Design review of the part built by this model. Coordinates are the model's own, in mm. Face numbers are marked on the shaded views. Coordinates: 2 decimals unless noted, no trailing zeros. Order: outer loops, then holes, each group sorted by start corner. A loop starts at its lowest first (then second) coordinate and runs counter-clockwise, first axis right, second up. Notation, with made-up numbers: (69.25, -19.5) -> (113.25, -19.5) arc R9 cw to (113.25, -15.5) -> close; hole circle Ø9 at (78.25, -7). An arc over 180 degrees is marked (long way). Use a Markdown table: item, result. Add a question column.
Q1. The part is to be moulded in two halves that separate along X. For the marked faces 1, 2 and 3, say which applies: pulls with the +X half, pulls with the -X half, needs draft (parallel to the pull), parting line crosses it, or undercut.
Q2. Insertion check: pin 1 (1 mm diameter, centred on x = -16.5, z = 7, fed in from +Y). The pin has a flat end and moves straight along its axis. Give the tip position at first contact, or say it passes through.
Q3. Add section C-C (x = 18.5). State the section outline as (y, z) points, then the cut area to 3 significant figures.
Q4. Wall thickness on probe 1 along Z at (x, y) = (-1, 6); probe 2 along X at (y, z) = (6.75, -32); probe 3 along Z at (x, y) = (-22.5, 0.75): over which ranges is each line inside the solid? List them lowest first.
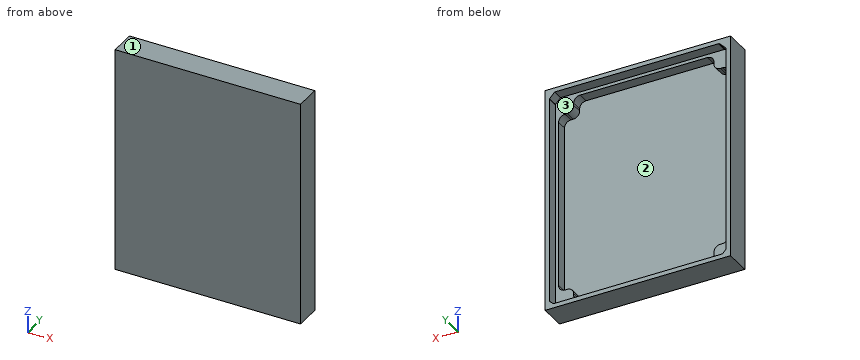
Autodesk Inventor part; units mm, degrees
ref_plane "YZ Plane" through (0, 0, 0) normal (1, 0, 0) x (0, 1, 0)
ref_plane "XZ Plane" through (0, 0, 0) normal (0, 1, 0) x (-1, 0, 0)
ref_plane "XY Plane" through (0, 0, 0) normal (0, 0, 1) x (1, 0, 0)
sketch "Sketch1" plane through (0, 0, 0) normal (0, 1, 0) x (-1, 0, 0)
  line L0 (41, 50.45) -> (40.9472, -50.4928) construction
  line L1 (40.9472, -50.4928) -> (-41, -50.45) construction
  line L2 (-41, -50.45) -> (-40.9472, 50.4928) construction
  line L3 (-40.9472, 50.4928) -> (41, 50.45) construction
  line L4 (-41, 50.45) -> (41, -50.45) construction
  line L5 (41, 50.45) -> (-41, -50.45) construction
  line L6 (-43, 52.45) -> (43, 52.45)
  line L7 (43, 52.45) -> (43, -52.45)
  line L8 (43, -52.45) -> (-43, -52.45)
  line L9 (-43, -52.45) -> (-43, 52.45)
  line L10 (-43, 52.45) -> (43, -52.45) construction
  line L11 (43, 52.45) -> (-43, -52.45) construction
  line L12 (41, 50.45) -> (41, 50.0105)
  line L13 (41.001, 46.9167) -> (41.001, -48.4427)
  line L14 (41, -50.45) -> (40.9473, -50.45)
  line L15 (39.0158, -50.4509) -> (-38.9625, -50.4509)
  line L16 (-38.3742, 50.45) -> (37.4278, 50.45)
  line L17 (-40.999, -48.5131) -> (-40.9487, 47.6278)
  line L18 (37.4278, 50.45) -> (37.7432, 50.4517)
  line L19 (41.001, 46.9167) -> (41.0014, 47.2908)
  line L20 (41.0014, 47.2908) -> (37.7432, 50.4517)
  line L21 (41.001, -48.4427) -> (41.001, -48.6823)
  line L22 (41.001, -48.6823) -> (39.229, -50.4509)
  line L23 (39.229, -50.4509) -> (39.0158, -50.4509)
  line L24 (-38.9625, -50.4509) -> (-39.191, -50.4509)
  line L25 (-39.191, -50.4509) -> (-40.9991, -48.7299)
  line L26 (-40.999, -48.5131) -> (-40.9991, -48.7299)
  line L27 (-40.9487, 47.6278) -> (-40.9486, 47.9339)
  line L28 (-38.3742, 50.45) -> (-38.6199, 50.45)
  line L29 (-38.6199, 50.45) -> (-40.9486, 47.9339)
  point P0 (0, 0)
  dimension "d48" = 82
  dimension "d49" = 100.9
  dimension "d50" = 86
  dimension "d51" = 104.9
extrude "Extrusion3" add sketch "Sketch1" along normal blind 10
sketch "Sketch3" plane through (0, 0, 0) normal (0, -1, 0) x (1, 0, 0)
  line L0 (43, -52.45) -> (-43, -52.45)
  line L1 (-43, 52.45) -> (43, 52.45)
  line L2 (43, 52.45) -> (43, -52.45)
  line L3 (43, -52.45) -> (-43, -52.45)
  line L4 (-43, -52.45) -> (-43, 52.45)
  line L5 (-43, 52.45) -> (43, -52.45) construction
  line L6 (43, 52.45) -> (-43, -52.45) construction
  point P0 (0, 0)
extrude "Extrusion4" add sketch "Sketch3" along normal blind 2
sketch "Sketch4" plane through (0, 0, 0) normal (0, 1, 0) x (1, 0, 0)
  line L0 (-40.966, -50.4517) -> (-40.966, 50.4509) construction
  line L1 (-40.966, 50.4509) -> (40.9486, 50.4509) construction
  line L2 (40.9486, 50.4509) -> (40.9486, -50.4517) construction
  line L3 (40.9486, -50.4517) -> (-40.966, -50.4517) construction
  line L4 (-41.001, -46.9167) -> (-41.001, 48.6823)
  line L5 (-37.7432, -50.4517) -> (-41.0014, -47.2908)
  line L6 (38.6199, -50.45) -> (-37.4278, -50.45)
  line L7 (43, 52.45) -> (-43, 52.45)
  line L8 (-43, 52.45) -> (-43, -52.45)
  line L9 (-43, -52.45) -> (43, -52.45)
  line L10 (43, -52.45) -> (43, 52.45)
  line L11 (-41.0014, -47.2908) -> (-41.001, -46.9167)
  line L12 (-41.001, -46.9167) -> (-41.001, 48.6823)
  line L13 (-41.001, 48.6823) -> (-39.229, 50.4509)
  line L14 (-39.229, 50.4509) -> (38.9625, 50.4509)
  line L15 (38.9625, 50.4509) -> (39.191, 50.4509)
  line L16 (39.191, 50.4509) -> (40.9991, 48.7299)
  line L17 (40.9991, 48.7299) -> (40.9486, -47.9339)
  line L18 (40.9486, -47.9339) -> (38.6199, -50.45)
  line L19 (38.6199, -50.45) -> (-37.4278, -50.45)
  line L20 (-37.4278, -50.45) -> (-37.7432, -50.4517)
  line L21 (-37.7432, -50.4517) -> (-41.0014, -47.2908)
  line L22 (-39.229, 50.4509) -> (38.9625, 50.4509)
  line L23 (-41.001, 48.6823) -> (-39.229, 50.4509)
  point P0 (0, 0)
sketch "Sketch5" plane through (0, 0, 0) normal (0, 1, 0) x (1, 0, 0)
  line L0 (-37.7432, -50.4517) -> (-41.0014, -47.2908)
  line L1 (-37.4278, -50.45) -> (-37.7432, -50.4517)
  line L2 (38.6199, -50.45) -> (-37.4278, -50.45)
  line L3 (40.9486, -47.9339) -> (38.6199, -50.45)
  line L4 (40.9991, 48.7299) -> (40.9486, -47.9339)
  line L5 (39.191, 50.4509) -> (40.9991, 48.7299)
  line L6 (38.9625, 50.4509) -> (39.191, 50.4509)
  line L7 (-39.229, 50.4509) -> (38.9625, 50.4509)
  line L8 (-41.001, 48.6823) -> (-39.229, 50.4509)
  line L9 (-41.001, -46.9167) -> (-41.001, 48.6823)
  line L10 (-41.0014, -47.2908) -> (-41.001, -46.9167)
  line L11 (-37.7432, -50.4517) -> (-41.0014, -47.2908)
  line L12 (38.6199, -50.45) -> (-37.4278, -50.45)
  line L13 (-37.4278, -50.45) -> (-37.7432, -50.4517)
  line L14 (-41.001, -46.9167) -> (-41.001, 48.6823)
  line L15 (-41.0014, -47.2908) -> (-41.001, -46.9167)
  line L16 (-41.001, 48.6823) -> (-39.229, 50.4509)
  line L17 (-39.229, 50.4509) -> (38.9625, 50.4509)
  line L18 (39.191, 50.4509) -> (40.9991, 48.7299)
  line L19 (40.9991, 48.7299) -> (40.9486, -47.9339)
  line L20 (40.9486, -47.9339) -> (38.6199, -50.45)
  line L21 (-41.0014, -47.2908) -> (-40.9669, 48.7164)
  line L22 (-39.229, 50.4509) -> (39.191, 50.4509)
  line L23 (40.9485, 48.778) -> (40.9486, -47.9339)
  line L24 (38.6199, -50.45) -> (-37.7432, -50.4517)
  line L25 (-37.7432, -50.4517) -> (-41.0014, -47.2908)
  line L26 (39.5283, -48.9788) -> (-39.5283, -48.9788)
  line L27 (-39.5283, -48.9788) -> (-39.5283, 48.9788)
  line L28 (-39.5283, 48.9788) -> (39.5283, 48.9788)
  line L29 (39.5283, 48.9788) -> (39.5283, -48.9788)
  line L30 (39.5283, -48.9788) -> (-39.5283, 48.9788) construction
  line L31 (-39.5283, -48.9788) -> (39.5283, 48.9788) construction
  line L32 (-39.5283, -48.9788) -> (-32.5283, -48.9788)
  line L33 (-32.5283, -48.9788) -> (-32.5283, -41.9788)
  line L34 (-32.5283, -41.9788) -> (-39.5283, -41.9788)
  line L35 (-39.5283, -41.9788) -> (-39.5283, -48.9788)
  line L36 (-39.5283, 48.9788) -> (-32.5283, 48.9788)
  line L37 (-32.5283, 48.9788) -> (-32.5283, 41.9788)
  line L38 (-32.5283, 41.9788) -> (-39.5283, 41.9788)
  line L39 (-39.5283, 41.9788) -> (-39.5283, 48.9788)
  line L40 (39.5283, 48.9788) -> (32.5283, 48.9788)
  line L41 (32.5283, 48.9788) -> (32.5283, 41.9788)
  line L42 (32.5283, 41.9788) -> (39.5283, 41.9788)
  line L43 (39.5283, 41.9788) -> (39.5283, 48.9788)
  line L44 (39.5283, -48.9788) -> (32.5283, -48.9788)
  line L45 (32.5283, -48.9788) -> (32.5283, -41.9788)
  line L46 (32.5283, -41.9788) -> (39.5283, -41.9788)
  line L47 (39.5283, -41.9788) -> (39.5283, -48.9788)
  point P0 (0, 0)
  point P1 (-41.001, -46.1517)
  point P2 (-39.5283, -48.7199)
  point P3 (-39.2615, -48.9788)
  dimension "d152" = 7
  dimension "d153" = 7
  dimension "d154" = 7
  dimension "d155" = 7
  dimension "d156" = 7
  dimension "d157" = 7
  dimension "d158" = 7
  dimension "d159" = 7
extrude "Extrusion5" add sketch "Sketch5" along normal blind 5 contours L0 L26 L29 L28 L27 L10 L21 L8 L7 L6 L5 L23 L3 L2 L1 | L0 L27 L34 L33 L26 | L45 L46 L29 L26 | L27 L28 L37 L38 | L42 L41 L28 L29
fillet "Fillet1" radius 3 12 edges at (-39.5283, 2.5, 41.9788) (-32.5283, 2.5, 41.9788) (-32.5283, 2.5, 48.9788) (-32.5283, 2.5, -48.9788) (-32.5283, 2.5, -41.9788) (-39.5283, 2.5, -41.9788) (32.5283, 2.5, -48.9788) (32.5283, 2.5, -41.9788) (39.5283, 2.5, -41.9788) (39.5283, 2.5, 41.9788) (32.5283, 2.5, 41.9788) (32.5283, 2.5, 48.9788)
properties part number "box"
Established:
| question | item | result |
|---|---|---|
| 1 | face 1 | needs draft |
| 1 | face 2 | undercut |
| 1 | face 3 | undercut |
| 2 | pin 1 | y = 0 |
| 3 | outline | (-2, -52.45) -> (10, -52.45) -> (10, -50.45) -> (5, -50.45) -> (5, -48.98) -> (0, -48.98) -> (0, 48.98) -> (5, 48.98) -> (5, 50.45) -> (10, 50.45) -> (10, 52.45) -> (-2, 52.45) -> close |
| 3 | area | 265 mm^2 |
| 4 | probe 1 | -52.45 to -50.45, 50.45 to 52.45 |
| 4 | probe 2 | -43 to -41, 40.99 to 43 |
| 4 | probe 3 | -52.45 to -48.98, 48.98 to 52.45 |
